from build123d import *

# Parameters (mm, degrees)
BOSS_EXTRUDE3_DEPTH = 3
BOSS_EXTRUDE4_DEPTH = 48
CUT_EXTRUDE1_REACH  = 53
SKETCH3_R           = 2.25


with BuildPart() as part:
    # Sketch1 → Boss-Extrude3 (new body)
    with BuildSketch(Plane(origin=(0, 0, 0), x_dir=(1, 0, 0), z_dir=(0, 1, 0))):
        with BuildLine():
            Line((0, 110), (0, 174))
            ThreePointArc((0, 174), (-160.755038657, 66.586917232), (-123.036579926, -123.036579926))
            Line((-123.036579926, -123.036579926), (-77.781745931, -77.781745931))
            ThreePointArc((-77.781745931, -77.781745931), (-101.626748576, 42.09517756), (0, 110))
        make_face()
    extrude(amount=BOSS_EXTRUDE3_DEPTH)

    # Sketch2 → Boss-Extrude4 (add)
    with BuildSketch(Plane(origin=(0, 3, 0), x_dir=(1, 0, 0), z_dir=(0, 1, 0))):
        with BuildLine():
            Line((0, 174), (-31.15408253, 105.496081168))
            ThreePointArc((-31.15408253, 105.496081168), (-33.083376151, 104.907055161), (-35.001544118, 104.282749817))
            Line((-35.001544118, 104.282749817), (-3.30998401, 173.96851441))
            ThreePointArc((-3.30998401, 173.96851441), (-1.655066878, 173.992128424), (0, 174))
        make_face()
        with BuildLine():
            Line((-109.065465459, 135.575529666), (-90.400634695, 62.671566494))
            ThreePointArc((-90.400634695, 62.671566494), (-91.534672677, 61.00330891), (-92.637928339, 59.31453644))
            Line((-92.637928339, 59.31453644), (-111.624769164, 133.476255975))
            ThreePointArc((-111.624769164, 133.476255975), (-110.350109434, 134.531978904), (-109.065465459, 135.575529666))
        make_face()
        with BuildLine():
            Line((-169.961014343, 37.272692462), (-109.720790239, -7.832508497))
            ThreePointArc((-109.720790239, -7.832508497), (-109.558712711, -9.843194048), (-109.359791534, -11.850569418))
            Line((-109.359791534, -11.850569418), (-170.639294189, 34.032797103))
            ThreePointArc((-170.639294189, 34.032797103), (-170.307858813, 35.654357748), (-169.961014343, 37.272692462))
        make_face()
        with BuildLine():
            Line((-155.791483302, -77.492023659), (-80.581598087, -74.877273253))
            ThreePointArc((-80.581598087, -74.877273253), (-79.194988304, -76.342346228), (-77.781745931, -77.781745931))
            Line((-77.781745931, -77.781745931), (-154.289169819, -80.441606627))
            ThreePointArc((-154.289169819, -80.441606627), (-155.047340737, -78.970387679), (-155.791483302, -77.492023659))
        make_face()
    extrude(amount=BOSS_EXTRUDE4_DEPTH)

    # Sketch3 → Cut-Extrude1 (cut, up to next)
    with BuildSketch(Plane.XZ, mode=Mode.PRIVATE) as cut_extrude1_sk1:
        with Locations((-57.053465335, -122.35155125)):
            Circle(SKETCH3_R)
    cut_extrude1_tool1 = extrude(cut_extrude1_sk1.sketch, amount=-CUT_EXTRUDE1_REACH, mode=Mode.PRIVATE) & part.part
    add(cut_extrude1_tool1.solids().sort_by_distance((-57.053465, 0, -122.351551))[0], mode=Mode.SUBTRACT)
    # Sketch3 → Cut-Extrude1 (cut, up to next)
    with BuildSketch(Plane.XZ, mode=Mode.PRIVATE) as cut_extrude1_sk2:
        with Locations((-130.399986549, 34.940571089)):
            Circle(SKETCH3_R)
    cut_extrude1_tool2 = extrude(cut_extrude1_sk2.sketch, amount=-CUT_EXTRUDE1_REACH, mode=Mode.PRIVATE) & part.part
    add(cut_extrude1_tool2.solids().sort_by_distance((-130.399987, 0, 34.940571))[0], mode=Mode.SUBTRACT)


solid = part.part
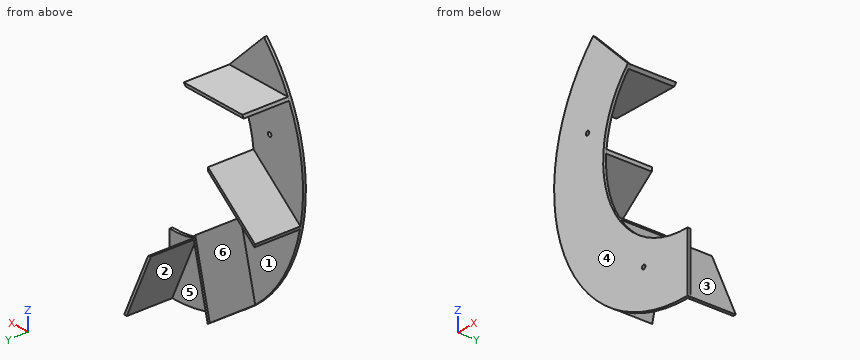
Source: CAD feature listing. Evaluate the final solid. Frame: model axes, mm. Face numbers are marked on the shaded views. A direction names the side the tool comes from. Round coordinates to 2 decimals unless told otherwise and drop trailing zeros. Order: outer loops, then holes, each group sorted by start corner. A loop starts at its lowest first (then second) coordinate and runs counter-clockwise, first axis right, second up. Notation, with made-up numbers: (-23.5, 8) - (-12.5, 8) arc R8 cw to (-12.5, 13) - close; hole circle Ø11 at (-31, 31.5). An arc over 180 degrees is marked (long way). Use a Markdown table: item, result. Add a question column.
1. Section query B-B (x = -99). Return the cut outline in (y, z).
2. Section query C-C (z = -12.5). Return the cut outline in (x, y).
3. Section query D-D (x = -147.5). Return the cut outline in (y, z), then the cut area to 3 significant figures.
4. Mould query, pull axis Z, two halves, no side actions, for the marked faces 1, 2 and 3. Classes: +Z half, -Z half, draft (parallel to the pull), parting line (faces both ways), or undercut.
5. Set-up query: the marked faces 4, 5 and 6. Return all of +Z, -Z, +X, -X, +Y, -Y with unobstructed straight access to the full face (end or side cutting, diameter ignored); none if empty.
6. First-contact query: pin 1 (10 mm diameter, centred on y = 17, z = -144, fed in from +X); pin 2 (5 mm diameter, centred on x = -130.4, z = 34.94, fed in from +Y); pin 3 (6 mm diameter, centred on y = 45.5, z = -0.5, fed in from +X); pin 4 (6 mm diameter, centred on x = -144.5, z = -13.5, fed in from -Y). Flat tips, straight axial feed; report the tip coordinate or a pass-through.
7. Section query A-A (y = 30.5). Return the cut outline in (x, z).
8. Line query: probe 1 along Z at (x, y) = (-78, 48.5); probe 2 along X at (y, z) = (29.5, -109); probe 3 along Y at (x, z) = (-155, -56). Output: solid intervals per line, ascending.
Derived:
| question | item | result |
|---|---|---|
| 1 | outline | (0, -143.09) - (3, -143.09) - (3, -96.26) - (51, -96.26) - (51, -84.16) - (3, -84.16) - (3, -47.95) - (0, -47.95) - close; (0, 47.95) - (3, 47.95) - (3, 75.52) - (51, 75.52) - (51, 78.52) - (3, 78.52) - (3, 99) - (0, 99) - close |
| 2 | outline | (-173.55, 0) - (-109.29, 0) - (-109.29, 3) - (-136.88, 3) - (-136.88, 51) - (-141.88, 51) - (-141.88, 3) - (-173.55, 3) - close |
| 3 | outline | (0, -92.3) - (3, -92.3) - (3, -20.45) - (51, -20.45) - (51, -16.71) - (3, -16.71) - (3, 77.2) - (51, 77.2) - (51, 80.21) - (3, 80.21) - (3, 92.3) - (0, 92.3) - close |
| 3 | area | 878 mm2 |
| 4 | face 1 | undercut |
| 4 | face 2 | -Z half |
| 4 | face 3 | +Z half |
| 5 | face 4 | +Z, -Z, +X, -X, -Y |
| 5 | face 5 | -Z, +Y |
| 5 | face 6 | -X, +Y |
| 6 | pin 1 | x = -11.37 |
| 6 | pin 2 | y = 3 |
| 6 | pin 3 | x = -116.84 |
| 6 | pin 4 | y = 0 |
| 7 | outline | (-170.64, -34.03) arc R174 ccw to (-169.96, -37.27) - (-109.72, 7.83) arc R110 cw to (-109.36, 11.85) - close; (-155.79, 77.49) - (-80.58, 74.88) arc R110 cw to (-77.78, 77.78) - (-154.29, 80.44) arc R174 ccw to start; (-111.62, -133.48) arc R174 ccw to (-109.07, -135.58) - (-90.4, -62.67) arc R110 cw to (-92.64, -59.31) - close; (-35, -104.28) - (-3.31, -173.97) arc R174 ccw to (0, -174) - (-31.15, -105.5) arc R110 cw to start |
| 8 | probe 1 | 77.56 to 77.79 |
| 8 | probe 2 | -105.36 to -102.26, -32.86 to -29.56 |
| 8 | probe 3 | 0 to 3 |
